```python
from build123d import *

# Parameters (mm, degrees)
MODEL_R             = 0.7834936
MODEL_R_2           = 6.5
MODEL_W             = 10.5
MODEL_H             = 3
MODEL_H_2           = 4
MODEL_R_3           = 1.229367
EXTRUDE_8_DEPTH     = 1.6
CUT_EXTRUDE_1_DEPTH = 10


with BuildPart() as part:
    # Model → 凸台-拉伸8 (new body)
    with BuildSketch(Plane.XY):
        with BuildLine():
            Line((-28.162112801, 27.669809042), (-37.212112801, 27.669809042))
            Line((-37.212112801, 27.669809042), (-37.212112801, -0.330212606))
            ThreePointArc((-37.212112801, -0.330212606), (-22.912101977, -14.630201782), (-8.612112801, -0.330190958))
            Line((-8.612112801, -0.330190958), (-8.612112801, 27.669809042))
            Line((-8.612112801, 27.669809042), (-17.662112801, 27.669809042))
            Line((-17.662112801, 27.669809042), (-17.662112801, 24.669809042))
            Line((-17.662112801, 24.669809042), (-16.932112801, 24.669809042))
            ThreePointArc((-16.932112801, 24.669809042), (-15.87145263, 24.230469214), (-15.432112801, 23.169809042))
            Line((-15.432112801, 23.169809042), (-15.432112801, -0.330190958))
            ThreePointArc((-15.432112801, -0.330190958), (-22.912112801, -7.810190958), (-30.392112801, -0.330190958))
            Line((-30.392112801, -0.330190958), (-30.392112801, 23.169809042))
            ThreePointArc((-30.392112801, 23.169809042), (-29.952772973, 24.230469214), (-28.892112801, 24.669809042))
            Line((-28.892112801, 24.669809042), (-28.162112801, 24.669809042))
            Line((-28.162112801, 24.669809042), (-28.162112801, 27.669809042))
        make_face()
        with Locations((-33.392112801, -0.330190958)):
            Circle(MODEL_R, mode=Mode.SUBTRACT)
        with Locations((-12.432112801, -0.330190958)):
            Circle(MODEL_R, mode=Mode.SUBTRACT)
        with Locations((-33.392112801, 24.669809042)):
            Circle(MODEL_R, mode=Mode.SUBTRACT)
        with Locations((-12.432112801, 24.669809042)):
            Circle(MODEL_R, mode=Mode.SUBTRACT)
        with BuildLine():
            Line((-30.392112801, -0.330190958), (-30.392112801, 23.169809042))
            ThreePointArc((-30.392112801, 23.169809042), (-29.952772973, 24.230469214), (-28.892112801, 24.669809042))
            Line((-28.892112801, 24.669809042), (-16.932112801, 24.669809042))
            ThreePointArc((-16.932112801, 24.669809042), (-15.87145263, 24.230469214), (-15.432112801, 23.169809042))
            Line((-15.432112801, 23.169809042), (-15.432112801, -0.330190958))
            ThreePointArc((-15.432112801, -0.330190958), (-22.912112801, -7.810190958), (-30.392112801, -0.330190958))
        make_face()
        with Locations((-22.912112801, -0.330190958)):
            Circle(MODEL_R_2, mode=Mode.SUBTRACT)
        with Locations((-22.912112801, 26.169809042)):
            Rectangle(MODEL_W, MODEL_H)
        with Locations((-22.912112801, 29.669809042)):
            Rectangle(MODEL_W, MODEL_H_2)
        with Locations((-22.912112801, 29.669809042)):
            Circle(MODEL_R_3, mode=Mode.SUBTRACT)
        with Locations((-22.912112801, 29.669809042)):
            Circle(MODEL_R_3)
        with Locations((-22.912112801, -0.330190958)):
            Circle(MODEL_R_2)
    extrude(amount=EXTRUDE_8_DEPTH)

    # 草图1 → 切除-拉伸1 (cut)
    with BuildSketch(Plane.XY.offset(1.6)):
        Polygon((-28.162112801, 27.669809042), (-17.662112801, 27.669809042), (-17.662112801, 34.986019155), (-28.743542957, 34.986019155), align=None)
    extrude(amount=-CUT_EXTRUDE_1_DEPTH, mode=Mode.SUBTRACT)


solid = part.part
```
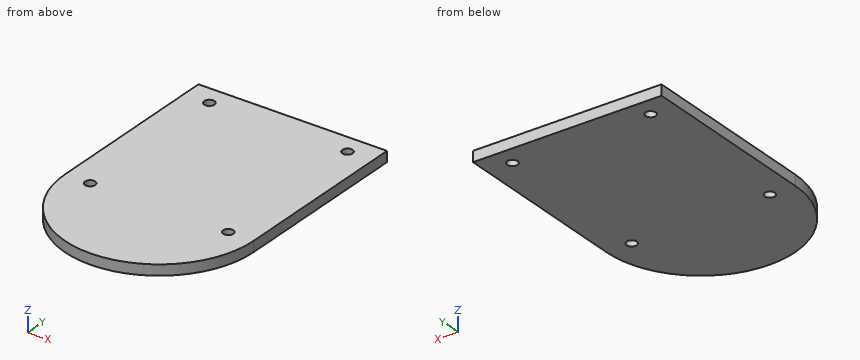
Model file for the job. Use its own axes, mm. Give positions to 0.01 mm unless a question says otherwise; leave off trailing zeros. Loops run counter-clockwise (first coordinate to the right, second up) from the corner with the lowest first, then second, coordinate; pieces in that order, holes last. Notation, with made-up numbers: (46.5, 15.5) -> (56.5, 15.5) arc R25 cw to (56.5, 45.5) -> close; hole circle Ø9 at (-28.5, -12.5). An arc over 180 degrees is marked (long way). Use CSV: the item, a comma, the result in double quotes. Start each with the question number.
1) Slice it at B-B on y = -5. Give the cut face in (x, z), plus the area to 3 significant figures.
2) Flat gauge pin, fed straight in: pin 1 Ø1.3 at (x, y) = (-33.39, 24.67) entering from +Z. Where does the tip first touch, or does it go through?
3) Slice it at C-C on x = -29. Give the cut face in (y, z), plus the area to 3 significant figures.
4) Slice it at A-A on z = 0.45. Give the cut face in (x, y), plus the area to 3 significant figures.
5) Wall check: line 1 (Y direction, x = -12.25, z = 0.5); line 2 (Y direction, x = -34, z = 0.85); line 3 (X direction, y = 24.5, z = 0.5). Give the ranges that are in metal, low to high.
Computed values:
1,outline,"(-36.43, 0) -> (-9.4, 0) -> (-9.4, 1.6) -> (-36.43, 1.6) -> close"
1,area,"43.3 mm^2"
2,pin 1,"passes through"
3,outline,"(-13.27, 0) -> (27.67, 0) -> (27.67, 1.6) -> (-13.27, 1.6) -> close"
3,area,"65.5 mm^2"
4,outline,"(-37.21, -0.33) arc R14.3 ccw to (-8.61, -0.33) -> (-8.61, 27.67) -> (-37.21, 27.67) -> close; hole circle Ø1.57 at (-33.39, -0.33); hole circle Ø1.57 at (-33.39, 24.67); hole circle Ø1.57 at (-12.43, -0.33); hole circle Ø1.57 at (-12.43, 24.67)"
4,area,"1,110 mm^2"
5,line 1,"y = -9.86 to -1.09, 0.43 to 23.91, 25.43 to 27.67"
5,line 2,"y = -9.36 to -0.82, 0.16 to 24.18, 25.16 to 27.67"
5,line 3,"x = -37.21 to -34.16, -32.63 to -13.2, -11.67 to -8.61"
